Drawing for the job (mm, zero at the part's lowest x, y, z). A direction names the side the tool comes from. Round coordinates to 2 decimals unless told otherwise and drop trailing zeros. Order: outer loops, then holes, each group sorted by start corner. A loop starts at its lowest first (then second) coordinate and runs counter-clockwise, first axis right, second up. Notation, with made-up numbers: (-18, -22) - (23, -22) arc R8 cw to (23, -13) - close; hole circle Ø6 at (-1, 71.25). An arc over 180 degrees is marked (long way). Answer as a JSON object with one key per item and string values.
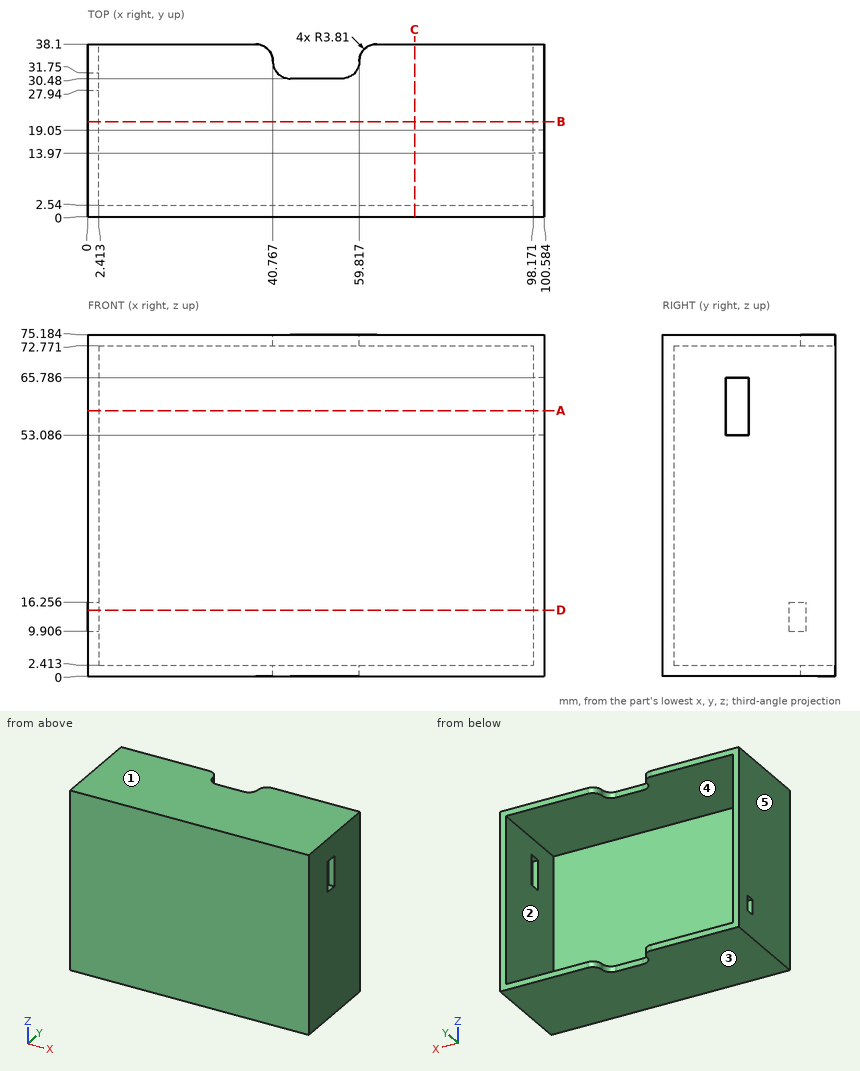
Item 1: Cut at C-C (x = 72). Write the cut outline in (y, z).
Taken from the geometry:
{"outline": "(0, 0) - (38.1, 0) - (38.1, 2.41) - (2.54, 2.41) - (2.54, 72.77) - (38.1, 72.77) - (38.1, 75.18) - (0, 75.18) - close"}
Item 2: Cut at D-D (z = 14.5). Write the cut outline in (x, y).
Taken from the geometry:
{"outline": "(0, 0) - (100.58, 0) - (100.58, 38.1) - (98.17, 38.1) - (98.17, 2.54) - (2.41, 2.54) - (2.41, 27.94) - (0, 27.94) - close; (0, 31.75) - (2.41, 31.75) - (2.41, 38.1) - (0, 38.1) - close"}
Item 3: Cut at B-B (y = 21). Write the cut outline in (x, z).
Taken from the geometry:
{"outline": "(0, 0) - (100.58, 0) - (100.58, 75.18) - (0, 75.18) - close; hole (2.41, 2.41) - (98.17, 2.41) - (98.17, 72.77) - (2.41, 72.77) - close"}
Item 4: Two-plate mould, pull along X, no slides. Class the marked faces 3, 4 and 5: pulls with the +X half, pulls with the -X half, needs draft (parallel to the pull), parting line crosses it, or undercut.
Taken from the geometry:
{"face 3": "needs draft", "face 4": "undercut", "face 5": "pulls with the -X half"}
Item 5: Cut at A-A (z = 58.5). Write the cut outline in (x, y), plus the area to 3 significant figures.
Taken from the geometry:
{"outline": "(0, 0) - (100.58, 0) - (100.58, 13.97) - (98.17, 13.97) - (98.17, 2.54) - (2.41, 2.54) - (2.41, 38.1) - (0, 38.1) - close; (98.17, 19.05) - (100.58, 19.05) - (100.58, 38.1) - (98.17, 38.1) - close", "area": "415 mm2"}
Item 6: Tool access for the marked faces 1 and 2: list every direction of +Z, -Z, +X, -X, +Y, -Y with a clear straight run to the whole face (end or side of a thin tool).
Taken from the geometry:
{"face 1": "+Z, +X, -X, +Y, -Y", "face 2": "+Y"}
Item 7: Drop flat-ended pins along their axis: P1, Ø2.5, axis at x = 53, z = 1, coming from the +Y side; P2, Ø5, axis at x = 88.5, z = 59, coming from the +Y side. Give the stop position or say it passes through.
Taken from the geometry:
{"P1": "y = 30.48", "P2": "y = 2.54"}
Item 8: Probe L1, parallel to X at y = 35, z = 50; L2, parallel to Z at x = 67, y = 14.5; L3, parallel to Y at x = 23, z = 53. List the from-to ranges inside material, lowest first. Write a range as from..to.
Taken from the geometry:
{"L1": "0..2.41, 98.17..100.58", "L2": "0..2.41, 72.77..75.18", "L3": "0..2.54"}
